```python
from build123d import *

# Parameters (mm, degrees)
CROQUIS1_W              = 44
CROQUIS1_H              = 78.5
SALIENTE_EXTRUIR1_DEPTH = 2
SALIENTE_EXTRUIR2_DEPTH = 12
CROQUIS3_W              = 44
CROQUIS3_H              = 78.5
SALIENTE_EXTRUIR3_DEPTH = 3.5
CROQUIS4_W              = 30.5
CROQUIS4_H              = 50
SALIENTE_EXTRUIR4_DEPTH = 2.5
CROQUIS6_W              = 12
CROQUIS6_H              = 14.873801133
CORTAR_EXTRUIR3_DEPTH   = 4
REDONDEO2_R             = 2
REDONDEO3_R             = 2
REDONDEO4_R             = 2
REDONDEO5_R             = 2
REDONDEO6_R             = 2


with BuildPart() as part:
    # Croquis1 → Saliente-Extruir1 (new body)
    # profile 1 of 2: a face of its own
    with BuildSketch(Plane.XY):
        with BuildLine():
            Line((45.934272818, 29.567618865), (45.934272818, 119.067618865))
            ThreePointArc((45.934272818, 119.067618865), (49.156098225, 126.845793458), (56.934272818, 130.067618865))
            Line((56.934272818, 130.067618865), (100.934272818, 130.067618865))
            ThreePointArc((100.934272818, 130.067618865), (108.712447411, 126.845793458), (111.934272818, 119.067618865))
            Line((111.934272818, 119.067618865), (111.934272818, 29.567618865))
            ThreePointArc((111.934272818, 29.567618865), (108.712447411, 21.789444272), (100.934272818, 18.567618865))
            Line((100.934272818, 18.567618865), (56.934272818, 18.567618865))
            ThreePointArc((56.934272818, 18.567618865), (49.156098225, 21.789444272), (45.934272818, 29.567618865))
        make_face()
        with BuildLine():
            ThreePointArc((56.934272818, 126.067618865), (51.98452535, 124.017366333), (49.934272818, 119.067618865))
            Line((49.934272818, 119.067618865), (49.934272818, 29.567618865))
            ThreePointArc((49.934272818, 29.567618865), (51.98452535, 24.617871397), (56.934272818, 22.567618865))
            Line((56.934272818, 22.567618865), (100.934272818, 22.567618865))
            ThreePointArc((100.934272818, 22.567618865), (105.884020287, 24.617871397), (107.934272818, 29.567618865))
            Line((107.934272818, 29.567618865), (107.934272818, 119.067618865))
            ThreePointArc((107.934272818, 119.067618865), (105.884020287, 124.017366333), (100.934272818, 126.067618865))
            Line((100.934272818, 126.067618865), (56.934272818, 126.067618865))
        make_face(mode=Mode.SUBTRACT)
    # profile 2 of 2: a face of its own
    with BuildSketch(Plane.XY):
        with BuildLine():
            Line((100.934272818, 126.067618865), (56.934272818, 126.067618865))
            ThreePointArc((56.934272818, 126.067618865), (51.98452535, 124.017366333), (49.934272818, 119.067618865))
            Line((49.934272818, 119.067618865), (49.934272818, 29.567618865))
            ThreePointArc((49.934272818, 29.567618865), (51.98452535, 24.617871397), (56.934272818, 22.567618865))
            Line((56.934272818, 22.567618865), (100.934272818, 22.567618865))
            ThreePointArc((100.934272818, 22.567618865), (105.884020287, 24.617871397), (107.934272818, 29.567618865))
            Line((107.934272818, 29.567618865), (107.934272818, 119.067618865))
            ThreePointArc((107.934272818, 119.067618865), (105.884020287, 124.017366333), (100.934272818, 126.067618865))
        make_face()
        with Locations((78.934272818, 68.817618865)):
            Rectangle(CROQUIS1_W, CROQUIS1_H, mode=Mode.SUBTRACT)
    extrude(amount=SALIENTE_EXTRUIR1_DEPTH)

    # Croquis2 → Saliente-Extruir2 (add)
    with BuildSketch(Plane.XY.offset(2)):
        with BuildLine():
            Line((100.934272818, 22.567618865), (56.934272818, 22.567618865))
            ThreePointArc((56.934272818, 22.567618865), (51.98452535, 24.617871397), (49.934272818, 29.567618865))
            Line((49.934272818, 29.567618865), (49.934272818, 115.941419998))
            Line((49.934272818, 115.941419998), (45.934272818, 115.941419998))
            Line((45.934272818, 115.941419998), (45.934272818, 29.567618865))
            ThreePointArc((45.934272818, 29.567618865), (49.156098225, 21.789444272), (56.934272818, 18.567618865))
            Line((56.934272818, 18.567618865), (100.934272818, 18.567618865))
            ThreePointArc((100.934272818, 18.567618865), (108.712447411, 21.789444272), (111.934272818, 29.567618865))
            Line((111.934272818, 29.567618865), (111.934272818, 115.941419998))
            Line((111.934272818, 115.941419998), (107.934272818, 115.941419998))
            Line((107.934272818, 115.941419998), (107.934272818, 29.567618865))
            ThreePointArc((107.934272818, 29.567618865), (105.884020287, 24.617871397), (100.934272818, 22.567618865))
        make_face()
    extrude(amount=SALIENTE_EXTRUIR2_DEPTH)

    # Croquis3 → Saliente-Extruir3 (add)
    # profile 1 of 4: a face of its own
    with BuildSketch(Plane.XY.offset(14)):
        with BuildLine():
            Line((45.934272818, 115.941419998), (49.934272818, 115.941419998))
            Line((49.934272818, 115.941419998), (49.934272818, 119.067618865))
            ThreePointArc((49.934272818, 119.067618865), (51.98452535, 124.017366333), (56.934272818, 126.067618865))
            Line((56.934272818, 126.067618865), (100.934272818, 126.067618865))
            ThreePointArc((100.934272818, 126.067618865), (105.884020287, 124.017366333), (107.934272818, 119.067618865))
            Line((107.934272818, 119.067618865), (107.934272818, 115.941419998))
            Line((107.934272818, 115.941419998), (111.934272818, 115.941419998))
            Line((111.934272818, 115.941419998), (111.934272818, 119.067618865))
            ThreePointArc((111.934272818, 119.067618865), (108.712447411, 126.845793458), (100.934272818, 130.067618865))
            Line((100.934272818, 130.067618865), (56.934272818, 130.067618865))
            ThreePointArc((56.934272818, 130.067618865), (49.156098225, 126.845793458), (45.934272818, 119.067618865))
            Line((45.934272818, 119.067618865), (45.934272818, 115.941419998))
        make_face()
    # profile 2 of 4: a face of its own
    with BuildSketch(Plane.XY.offset(14)):
        with BuildLine():
            Line((107.934272818, 115.941419998), (107.934272818, 29.567618865))
            ThreePointArc((107.934272818, 29.567618865), (105.884020287, 24.617871397), (100.934272818, 22.567618865))
            Line((100.934272818, 22.567618865), (56.934272818, 22.567618865))
            ThreePointArc((56.934272818, 22.567618865), (51.98452535, 24.617871397), (49.934272818, 29.567618865))
            Line((49.934272818, 29.567618865), (49.934272818, 115.941419998))
            Line((49.934272818, 115.941419998), (45.934272818, 115.941419998))
            Line((45.934272818, 115.941419998), (45.934272818, 29.567618865))
            ThreePointArc((45.934272818, 29.567618865), (49.156098225, 21.789444272), (56.934272818, 18.567618865))
            Line((56.934272818, 18.567618865), (100.934272818, 18.567618865))
            ThreePointArc((100.934272818, 18.567618865), (108.712447411, 21.789444272), (111.934272818, 29.567618865))
            Line((111.934272818, 29.567618865), (111.934272818, 115.941419998))
            Line((111.934272818, 115.941419998), (107.934272818, 115.941419998))
        make_face()
    # profile 3 of 4: a face of its own
    with BuildSketch(Plane.XY.offset(14)):
        with BuildLine():
            ThreePointArc((49.934272818, 29.567618865), (51.98452535, 24.617871397), (56.934272818, 22.567618865))
            Line((56.934272818, 22.567618865), (100.934272818, 22.567618865))
            ThreePointArc((100.934272818, 22.567618865), (105.884020287, 24.617871397), (107.934272818, 29.567618865))
            Line((107.934272818, 29.567618865), (107.934272818, 115.941419998))
            Line((107.934272818, 115.941419998), (107.934272818, 119.067618865))
            ThreePointArc((107.934272818, 119.067618865), (105.884020287, 124.017366333), (100.934272818, 126.067618865))
            Line((100.934272818, 126.067618865), (56.934272818, 126.067618865))
            ThreePointArc((56.934272818, 126.067618865), (51.98452535, 124.017366333), (49.934272818, 119.067618865))
            Line((49.934272818, 119.067618865), (49.934272818, 115.941419998))
            Line((49.934272818, 115.941419998), (49.934272818, 29.567618865))
        make_face()
        with Locations((78.934272818, 68.817618865)):
            Rectangle(CROQUIS3_W, CROQUIS3_H, mode=Mode.SUBTRACT)
    # profile 4 of 4: a face of its own
    with BuildSketch(Plane.XY.offset(14)):
        with Locations((78.934272818, 68.817618865)):
            Rectangle(CROQUIS3_W, CROQUIS3_H)
    extrude(amount=SALIENTE_EXTRUIR3_DEPTH)

    # Croquis4 → Saliente-Extruir4 (add)
    with BuildSketch(Plane.XY.offset(17.5)):
        Polygon((59.684272818, 103.317618865), (59.684272818, 99.317618865), (59.684272818, 45.317618865), (98.184272818, 45.317618865), (98.184272818, 103.317618865), align=None)
        with Locations((78.934272818, 74.317618865)):
            Rectangle(CROQUIS4_W, CROQUIS4_H, mode=Mode.SUBTRACT)
    extrude(amount=SALIENTE_EXTRUIR4_DEPTH)

    # Croquis6 → Cortar-Extruir3 (cut)
    with BuildSketch(Plane.ZY.offset(-45.934272818)):
        with Locations((8, 108.504519432)):
            Rectangle(CROQUIS6_W, CROQUIS6_H)
    extrude(amount=-CORTAR_EXTRUIR3_DEPTH, mode=Mode.SUBTRACT)

    # Redondeo2
    redondeo2_edges = [part.edges().sort_by_distance(p)[0] for p in [
        (78.934272818, 18.567618865, 0),
        (108.712447411, 21.789444272, 0),
        (111.934272818, 74.317618865, 0),
        (108.712447411, 126.845793458, 0),
        (78.934272818, 130.067618865, 0),
        (49.156098225, 126.845793458, 0),
        (45.934272818, 74.317618865, 0),
        (49.156098225, 21.789444272, 0),
    ]]
    fillet(redondeo2_edges, radius=REDONDEO2_R - 0.0001)  # a hair under: the kernel refuses the full size

    # Redondeo3
    redondeo3_edges = [part.edges().sort_by_distance(p)[0] for p in [
        (45.934272818, 74.317618865, 17.5),
        (78.934272818, 130.067618865, 17.5),
        (49.156098225, 21.789444272, 17.5),
        (78.934272818, 18.567618865, 17.5),
        (108.712447411, 21.789444272, 17.5),
        (111.934272818, 74.317618865, 17.5),
        (108.712447411, 126.845793458, 17.5),
        (49.156098225, 126.845793458, 17.5),
    ]]
    fillet(redondeo3_edges, radius=REDONDEO3_R)

    # Redondeo4
    redondeo4_edges = [part.edges().sort_by_distance(p)[0] for p in [
        (59.684272818, 74.317618865, 20),
        (78.934272818, 45.317618865, 20),
        (98.184272818, 74.317618865, 20),
        (78.934272818, 103.317618865, 20),
    ]]
    fillet(redondeo4_edges, radius=REDONDEO4_R)

    # Redondeo5
    redondeo5_edges = [part.edges().sort_by_distance(p)[0] for p in [
        (45.934272818, 101.067618865, 8),
    ]]
    fillet(redondeo5_edges, radius=REDONDEO5_R)

    # Redondeo6
    redondeo6_edges = [part.edges().sort_by_distance(p)[0] for p in [
        (111.934272818, 115.941419998, 8),
    ]]
    fillet(redondeo6_edges, radius=REDONDEO6_R)


solid = part.part
```
Work out the finished part from the listing and answer in its coordinate system (mm). A direction names the side the tool comes from. Give positions to 0.01 mm unless a question says otherwise; leave off trailing zeros. Loops run counter-clockwise (first coordinate to the right, second up) from the corner with the lowest first, then second, coordinate; pieces in that order, holes last. Notation, with made-up numbers: (-23.5, 67) - (-0.5, 67) arc R15 ccw to (-0.5, 96) - close; hole circle Ø3 at (4, 16.5). An arc over 180 degrees is marked (long way). One line per question, with ' | ' between items.
(1) The part is cut by section B-B (z = 11). Write down the section's boundary in (x, y).
Recorded:
outline: (45.93, 29.57) arc R11 ccw to (56.93, 18.57) - (100.93, 18.57) arc R11 ccw to (111.93, 29.57) - (111.93, 113.94) arc R2 ccw to (109.93, 115.94) - (107.93, 115.94) - (107.93, 29.57) arc R7 cw to (100.93, 22.57) - (56.93, 22.57) arc R7 cw to (49.93, 29.57) - (49.93, 101.07) - (47.93, 101.07) arc R2 ccw to (45.93, 99.07) - close
(2) The part is cut by section C-C (y = 52). Write down the section's boundary in (x, z).
Recorded:
outline: (45.93, 2) arc R2 ccw to (47.93, 0) - (56.93, 0) - (56.93, 2) - (49.93, 2) - (49.93, 14) - (107.93, 14) - (107.93, 2) - (100.93, 2) - (100.93, 0) - (109.93, 0) arc R2 ccw to (111.93, 2) - (111.93, 15.5) arc R2 ccw to (109.93, 17.5) - (98.18, 17.5) - (98.18, 18) arc R2 ccw to (96.18, 20) - (94.18, 20) - (94.18, 17.5) - (63.68, 17.5) - (63.68, 20) - (61.68, 20) arc R2 ccw to (59.68, 18) - (59.68, 17.5) - (47.93, 17.5) arc R2 ccw to (45.93, 15.5) - close
(3) The mould has two halves that part along Y. Classify faces 1 (the face through (106, 87, 0)), 2 (the face through (108.8, 126.76, 14.74)), 3 (the face through (79, 99.318, 19)), 4 (the face through (79, 29.568, 1)): +Y half, -Y half, draft (parallel to the pull), parting line (faces both ways), or undercut.
Recorded:
face 1: draft | face 2: +Y half | face 3: undercut | face 4: undercut
(4) A tool of negligible diameter and unlimited length cuts with its end or side. For faces 5 (the face through (111.4, 115.3, 8.1)), 6 (the face through (78, 77, 14)), 7 (the face through (109, 115.941, 8)), from which of +Z, -Z, +X, -X, +Y, -Y can it reach the whole face along a straight path? Write none if from no direction.
Recorded:
face 5: +X, +Y | face 6: +Y | face 7: +X, -X, +Y
(5) Straight lines are drawn through the part: probe 1 along Z at (x, y) = (54.5, 28.5); probe 2 along X at (y, z) = (88.5, 13); probe 3 along Z at (x, y) = (79.5, 74.5). For each, find the intervals that lie inside material, in ascending order.
Recorded:
probe 1: z = 0 to 2, 14 to 17.5 | probe 2: x = 45.93 to 49.93, 107.93 to 111.93 | probe 3: z = 14 to 17.5
(6) Each of these flat-tipped pins is pushed along its axis until it touches: pin 1 Ø0.6 at (y, z) = (71, 1) entering from +X; pin 2 Ø1 at (x, z) = (86, 1) entering from -Y; pin 3 Ø0.8 at (y, z) = (70.5, 18.5) entering from +X. Where does it stop, or does it pass through?
Recorded:
pin 1: stops at x = 111.81 | pin 2: stops at y = 18.63 | pin 3: stops at x = 98.18
